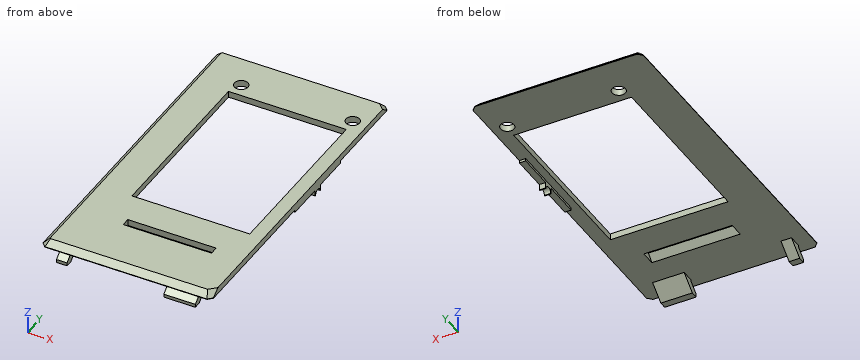
```python
from build123d import *

# Parameters (mm, degrees)
PAD014_DEPTH       = 1.5
SKETCH020_W        = 2.5
SKETCH020_H        = 5.25
SKETCH020_W_2      = 7.5
PAD015_DEPTH       = 3
POCKET012015_DEPTH = 36.751
SKETCH024_R        = 1.6
POCKET012016_DEPTH = 4.501
SKETCH026_W        = 21
SKETCH026_H        = 2
POCKET012017_DEPTH = 4.501
POCKET012018_DEPTH = 21
SKETCH038_W        = 28
SKETCH038_H        = 42
POCKET012019_DEPTH = 1.501
PAD017_DEPTH       = 1.5
CHAMFER001_SIZE    = 1.4


with BuildPart() as part:
    # Sketch016 → Pad014 (new body)
    with BuildSketch(Plane.XY.offset(13.5)):
        Polygon((-19.25, 38.75), (19.25, 38.75), (20.25, 37.75), (20.25, -37.75), (19.25, -38.75), (-19.25, -38.75), (-20.25, -37.75), (-20.25, 37.75), align=None)
    extrude(amount=PAD014_DEPTH)

    # Sketch020 → Pad015 (new body)
    with BuildSketch(Plane(origin=(0, 0, 13.5), x_dir=(1, 0, 0), z_dir=(0, 0, -1))):
        with Locations((-15.25, 36.125)):
            Rectangle(SKETCH020_W, SKETCH020_H)
        with Locations((12.75, 36.125)):
            Rectangle(SKETCH020_W_2, SKETCH020_H)
    extrude(amount=PAD015_DEPTH)

    # Sketch021 → Pocket012015 (cut, through all)
    with BuildSketch(Plane(origin=(-16.5, 0, 13.5), x_dir=(0, -1, 0), z_dir=(-1, 0, 0))):
        Polygon((36.5, 0), (38.75, 0), (38.75, -2.25), (36.5, -0.362026), align=None)
        Polygon((33.5, 0), (37.075261, -3), (33.5, -3), align=None)
    extrude(amount=-POCKET012015_DEPTH, mode=Mode.SUBTRACT)

    # Sketch024 → Pocket012016 (cut, through all)
    with BuildSketch(Plane.XY.offset(15)):
        with Locations((-9.75, 29.25)):
            Circle(SKETCH024_R)
        with Locations((16.75, 29.25)):
            Circle(SKETCH024_R)
    extrude(amount=-POCKET012016_DEPTH, mode=Mode.SUBTRACT)

    # Sketch026 → Pocket012017 (cut, through all)
    with BuildSketch(Plane.XY.offset(15)):
        with Locations((2.75, -24.75)):
            Rectangle(SKETCH026_W, SKETCH026_H)
    extrude(amount=-POCKET012017_DEPTH, mode=Mode.SUBTRACT)

    # Sketch027 → Pocket012018 (cut)
    with BuildSketch(Plane(origin=(13.25, 0, 13.5), x_dir=(0, -1, 0), z_dir=(-1, 0, 0))):
        Polygon((25.75, 1.5), (27.25, 0), (25.75, 0), align=None)
    extrude(amount=POCKET012018_DEPTH, mode=Mode.SUBTRACT)

    # Sketch038 → Pocket012019 (cut, through all)
    with BuildSketch(Plane(origin=(0, 0, 13.5), x_dir=(1, 0, 0), z_dir=(0, 0, -1))):
        with Locations((3, -5)):
            Rectangle(SKETCH038_W, SKETCH038_H)
    extrude(amount=-POCKET012019_DEPTH, mode=Mode.SUBTRACT)

    # Sketch040 → Pad017 (new body)
    with BuildSketch(Plane(origin=(20.25, 0, 13.5), x_dir=(0, 1, 0), z_dir=(1, 0, 0))):
        with BuildLine():
            Line((17.6, 0), (-2.2, 0))
            Line((-2.2, 0), (-2.2, -0.6))
            Line((-2.2, -0.6), (6.5, -0.6))
            Line((6.5, -0.6), (6.5, -2))
            Line((6.5, -2), (6.7, -2))
            ThreePointArc((8.7, -2), (7.7, -1), (6.7, -2))
            Line((8.9, -2), (8.7, -2))
            Line((8.9, -0.6), (8.9, -2))
            Line((8.9, -0.6), (17.6, -0.6))
            Line((17.6, -0.6), (17.6, 0))
        make_face()
    extrude(amount=-PAD017_DEPTH)

    # Chamfer001
    chamfer001_edges = [part.edges().sort_by_distance(p)[0] for p in [
        (19.75, 38.25, 15),
        (0, 38.75, 15),
        (-19.75, 38.25, 15),
        (-20.25, 0, 15),
        (-19.75, -38.25, 15),
        (0, -38.75, 15),
        (19.75, -38.25, 15),
    ]]
    chamfer(chamfer001_edges, length=CHAMFER001_SIZE)


solid = part.part
```
Design review of the part built by this model. Coordinates are the model's own, in mm. Give positions to 0.01 mm unless a question says otherwise; leave off trailing zeros. Order: outer loops, then holes, each group sorted by start corner. A loop starts at its lowest first (then second) coordinate and runs counter-clockwise, first axis right, second up. Notation, with made-up numbers: (-2, -27.75) - (17, -27.75) arc R31 ccw to (17, -1.75) - close; hole circle Ø9 at (41.25, 14). An arc over 180 degrees is marked (long way). Use a Markdown table: item, result. Add a question column.
(1) Wall thickness on probe 1 along Y at (x, z) = (16.75, 14.3); probe 2 along Y at (x, z) = (-9.75, 14.45); probe 3 along Z at (x, y) = (8, -23): over which ranges is each line inside the solid? List them lowest first. Write a range as [from, to].
(2) Add section D-D on y = 7.7. Give the boundary of the cut face in (x, z).
(3) Add section B-B on x = 14. Give the boundary of the cut face in (y, z), then the cut area to 3 significant figures.
(4) Add section A-A on y = 29.25. Give the boundary of the cut face in (x, z).
(5) Add section C-C on x = -7. Give the boundary of the cut face in (y, z), then the cut area to 3 significant figures.
(6) Clearance check with flat-ended pins moving along their axes: P1, Ø0.9, axis at y = -37, z = 12.5, coming from the -X side; P2, Ø1.1, axis at x = 19.5, z = 12, coming from the -Y side; P3, Ø0.9, axis at y = -36.5, z = 12.5, coming from the +X side. State where each tip first meets the part, or that it passes through.
Report:
| question | item | result |
|---|---|---|
| 1 | probe 1 | y = [-38.05, -16], [26, 27.65], [30.85, 38.05] |
| 1 | probe 2 | y = [-37.9, -16], [26, 27.65], [30.85, 37.9] |
| 1 | probe 3 | z = [13.5, 15] |
| 2 | outline | (-20.25, 13.5) - (-11, 13.5) - (-11, 15) - (-18.85, 15) - (-20.25, 13.6) - close; (17, 13.5) - (18.75, 13.5) - (18.75, 12.5) - (20.25, 12.5) - (20.25, 15) - (17, 15) - close |
| 3 | outline | (-38.75, 10.5) - (-37.08, 10.5) - (-33.5, 13.5) - (-16, 13.5) - (-16, 15) - (-37.35, 15) - (-38.75, 13.6) - (-38.75, 13.5) - (-36.5, 13.5) - (-36.5, 13.14) - (-38.75, 11.25) - close; (26, 13.5) - (38.75, 13.5) - (38.75, 13.6) - (37.35, 15) - (26, 15) - close |
| 3 | area | 58.7 mm² |
| 4 | outline | (-20.25, 13.5) - (-11.35, 13.5) - (-11.35, 15) - (-18.85, 15) - (-20.25, 13.6) - close; (-8.15, 13.5) - (15.15, 13.5) - (15.15, 15) - (-8.15, 15) - close; (18.35, 13.5) - (20.25, 13.5) - (20.25, 15) - (18.35, 15) - close |
| 5 | outline | (-38.75, 13.5) - (-27.25, 13.5) - (-25.75, 15) - (-37.35, 15) - (-38.75, 13.6) - close; (-23.75, 13.5) - (-16, 13.5) - (-16, 15) - (-23.75, 15) - close; (26, 13.5) - (38.75, 13.5) - (38.75, 13.6) - (37.35, 15) - (26, 15) - close |
| 5 | area | 47.2 mm² |
| 6 | P1 | stops at x = -16.5 |
| 6 | P2 | stops at y = 6.5 |
| 6 | P3 | stops at x = 16.5 |
